from build123d import *

# Parameters (mm, degrees)
SKETCH2_R             = 110
BOSS_EXTRUDE8_DEPTH   = 190
BOSS_EXTRUDE8_2_DEPTH = 190
BOSS_EXTRUDE9_DEPTH   = 640
SKETCH2_14_W          = 510.000000001
SKETCH2_14_H          = 380
BOSS_EXTRUDE10_DEPTH  = 130
BOSS_EXTRUDE11_REACH  = 1328.721


with BuildPart() as part:
    # Sketch2 → Boss-Extrude8 (new body)
    with BuildSketch(Plane(origin=(0, 0, 0), x_dir=(1, 0, 0), z_dir=(0, 1, 0))):
        with BuildLine():
            Line((317.819938748, -286.794238497), (-322.180061253, -286.794238497))
            Line((-322.180061253, -286.794238497), (-322.180061253, -573.39160802))
            ThreePointArc((-322.180061253, -573.39160802), (-2.180061253, -893.39160802), (317.819938748, -573.39160802))
            Line((317.819938748, -573.39160802), (317.819938748, -286.794238497))
        make_face()
        with Locations(Location((-2.180061253, -573.39160802, 0), (0, 0, 270))):
            Circle(SKETCH2_R, mode=Mode.SUBTRACT)
    extrude(amount=BOSS_EXTRUDE8_DEPTH)



with BuildPart() as body_2:
    # Sketch2 → Boss-Extrude8 2 (new body)
    with BuildSketch(Plane(origin=(0, 0, 0), x_dir=(1, 0, 0), z_dir=(0, 1, 0))):
        with BuildLine():
            ThreePointArc((317.819938748, 566.60839198), (-2.180061253, 886.60839198), (-322.180061253, 566.60839198))
            Line((-322.180061253, 566.60839198), (-322.180061253, 353.205761503))
            Line((-322.180061253, 353.205761503), (317.819938748, 353.205761503))
            Line((317.819938748, 353.205761503), (317.819938748, 566.60839198))
        make_face()
        with Locations(Location((-2.180061253, 566.60839198, 0), (0, 0, 270))):
            Circle(SKETCH2_R, mode=Mode.SUBTRACT)
    extrude(amount=BOSS_EXTRUDE8_2_DEPTH)


with BuildPart() as part_1:
    add(part.part)

    add(body_2.part)  # Boss-Extrude9 merges body 2
    # Sketch2_13 → Boss-Extrude9 (add)
    with BuildSketch(Plane(origin=(0, 0, 0), x_dir=(1, 0, 0), z_dir=(0, 1, 0))):
        Polygon((317.819938748, 353.205761503), (-322.180061253, 353.205761503), (-322.180061253, -286.794238497), (317.819938748, -286.794238497), (317.819938748, -156.794238497), (-192.180061253, -156.794238497), (-192.180061253, 223.205761503), (317.819938748, 223.205761503), align=None)
    extrude(amount=BOSS_EXTRUDE9_DEPTH)

    # Sketch2_14 → Boss-Extrude10 (add)
    with BuildSketch(Plane(origin=(0, 0, 0), x_dir=(1, 0, 0), z_dir=(0, 1, 0))):
        with Locations((62.819938748, 33.205761503)):
            Rectangle(SKETCH2_14_W, SKETCH2_14_H)
    extrude(amount=BOSS_EXTRUDE10_DEPTH)

    # Sketch13 → Boss-Extrude11 (add, up to next)
    with BuildSketch(Plane.XY.offset(-223.205761503), mode=Mode.PRIVATE) as boss_extrude11_sk1:
        Polygon((-192.180061253, 640), (317.819938748, 130), (-192.180061253, 130), align=None)
    boss_extrude11_tool1 = extrude(boss_extrude11_sk1.sketch, amount=BOSS_EXTRUDE11_REACH, mode=Mode.PRIVATE) - part_1.part
    add(boss_extrude11_tool1.solids().sort_by_distance((-22.180061, 300, -223.205762))[0])


solid = part_1.part
Design review of the part built by this model. Coordinates are the model's own, in mm. A direction names the side the tool comes from. Coordinates: 2 decimals unless noted, no trailing zeros. Order: outer loops, then holes, each group sorted by start corner. A loop starts at its lowest first (then second) coordinate and runs counter-clockwise, first axis right, second up. Notation, with made-up numbers: (58.5, 73.5) - (108.5, 73.5) arc R25 ccw to (108.5, 88.5) - close; hole circle Ø4 at (-29.5, 32). An arc over 180 degrees is marked (long way). Put each result on its own line as item: value.
1) Take a section at A-A, the plane z = -485. Give the boundary of the cut face in (x, y), and give its area (3 significant figures).
Response values:
outline: (-322.18, 0) - (-75.94, 0) - (-75.94, 190) - (-322.18, 190) - close; (71.58, 0) - (317.82, 0) - (317.82, 190) - (71.58, 190) - close
area: 93,600 mm²
2) Insertion check: P1, Ø1.5, axis at x = -38, y = 283.5, coming from the -Z side; P2, Ø3, axis at x = 52.5, z = -425, coming from the +Y side. Each pin has a flat end and moves straight along its axis. Give the tip position at first contact, or say it passes through.
Response values:
P1: stops at z = -353.21
P2: stops at y = 190
3) Take a section at C-C, the plane z = -112.5. Give the boundary of the cut face in (x, y), and give its area (3 significant figures).
Response values:
outline: (-322.18, 0) - (317.82, 0) - (317.82, 130) - (-192.18, 640) - (-322.18, 640) - close
area: 280,000 mm²
4) The part is to be moulded in two halves that separate along X. For faces 1 (the face through (4.86, 93.67, -886.53)), 2 (the face through (317.82, 102, 11)), 3 (the face through (-69.113, 93.67, -653.901)), 4 (the face through (2, 412, -353.206)), say which applies: released by +X, released by -X, zero draft, split by the parting line, or undercut.
Response values:
face 1: split by the parting line
face 2: released by +X
face 3: undercut
face 4: zero draft
5) Wall thickness on L1, parallel to Z at x = 100, y = 444; L2, parallel to Y at x = -186, z = -459; L3, parallel to Z at x = 173.5, y = 260: over which ranges is each line inside the solid? List them lowest first. Write a range as from..to.
Response values:
L1: z = -353.21..-223.21, 156.79..286.79
L2: y = 0..190
L3: z = -353.21..286.79
6) Tool access review of faces 5 (the face through (-7, 190, -683)), 6 (the face through (180, 495, 156.794)), 7 (the face through (-7, 190, 451)), 8 (the face through (-220, 640, -38)), 9 (the face through (-7, 0, -9)): name each direction out of +Z, -Z, +X, -X, +Y, -Y from which nothing blocks a thin tool from reaching the whole face with its end or side.
Response values:
face 5: -Z, +X, -X, +Y
face 6: +X, +Y
face 7: +Z, +X, -X, +Y
face 8: +Z, -Z, +X, -X, +Y
face 9: +Z, -Z, +X, -X, -Y
7) Take a section at B-B, the plane x = 42.5. Give the boundary of the cut face in (y, z).
Response values:
outline: (0, -883.47) - (190, -883.47) - (190, -667.13) - (0, -667.13) - close; (0, -466.09) - (190, -466.09) - (190, -353.21) - (640, -353.21) - (640, -223.21) - (405.32, -223.21) - (405.32, 156.79) - (640, 156.79) - (640, 286.79) - (190, 286.79) - (190, 472.87) - (0, 472.87) - close; (0, 673.91) - (190, 673.91) - (190, 890.26) - (0, 890.26) - close
8) Take a section at D-D, the plane y = 595. Give the boundary of the cut face in (x, z).
Response values:
outline: (-322.18, -353.21) - (317.82, -353.21) - (317.82, -223.21) - (-147.18, -223.21) - (-147.18, 156.79) - (317.82, 156.79) - (317.82, 286.79) - (-322.18, 286.79) - close
